For this review, use the dimensioned drawing (mm, ordinates from the lowest corner) and the shaded views. A direction names the side the tool comes from. Give positions to 0.01 mm unless a question says otherwise; leave off trailing zeros. Order: outer loops, then holes, each group sorted by start corner. A loop starts at its lowest first (then second) coordinate and runs counter-clockwise, first axis right, second up. Notation, with made-up numbers: M 20,55 L 47,55 A17 cw 47,77 Z; hole C 59.25,0.5 d3. An arc over 180 degrees is marked long. Answer as CSV lines item,"result". Start each with the question number.
1. We need section D-D, the plane y = 8. Give the boundary of the cut face in (x, z).
2. Clearance check with flat-ended pins moving along their axes: P1, Ø2, axis at x = 8, z = 16, coming from the -Y side; P2, Ø2, axis at y = 7.5, z = 30, coming from the -X side; P3, Ø1.5, axis at x = 3.5, z = 27.5, coming from the -Y side. State where each tip first meets the part, or that it passes through.
3. We need section C-C, the plane z = 19. Give the boundary of the cut face in (x, y).
4. For line 1 along Z through (x, y) = (6.5, 5); line 2 along Z through (x, y) = (1, 3.5); line 3 along X through (y, z) = (8.5, 22.5), list the stretches that pass through material, from the lowest coordinate up.
5. We need section A-A, the plane y = 5. Give the boundary of the cut face in (x, z), and give its area (3 significant figures).
6. Machinability: for the marked faces 1 and 2, which of the approach directions +Z, -Z, +X, -X, +Y, -Y give a long, thin tool a straight path to every point of the face, cutting with its end or side? Answer none if there is none.
7. We need section B-B, the plane x = 5. Give the boundary of the cut face in (y, z).
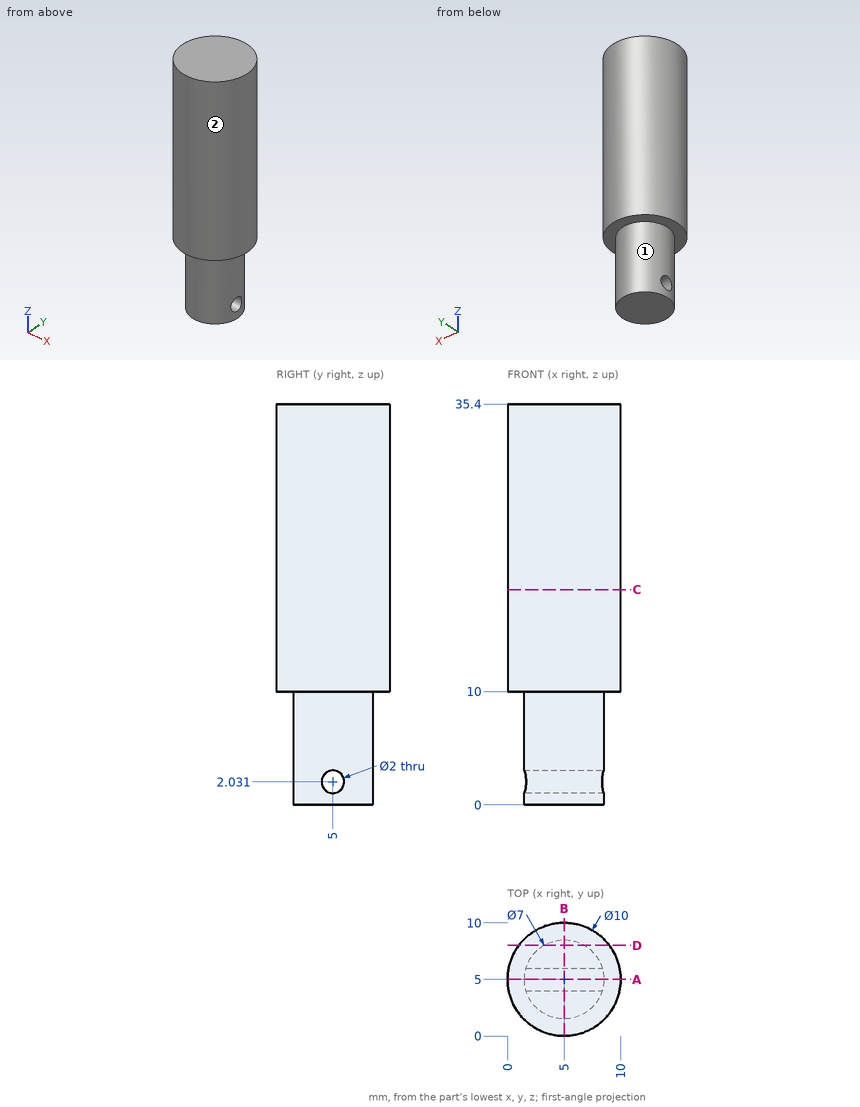
Result set:
1,outline,"M 1,10 L 3.2,10 L 3.2,0 L 6.8,0 L 6.8,10 L 9,10 L 9,35.4 L 1,35.4 Z"
2,P1,"y = 0.42"
2,P2,"x = 0.23"
2,P3,"y = 0.06"
3,outline,"C 5,5 d10"
4,line 1,"0 to 1.03, 3.03 to 35.4"
4,line 2,"10 to 35.4"
4,line 3,"1.43 to 8.57"
5,outline,"M 0,10 L 1.5,10 L 1.5,3.03 L 8.5,3.03 L 8.5,10 L 10,10 L 10,35.4 L 0,35.4 Z; M 1.5,0 L 8.5,0 L 8.5,1.03 L 1.5,1.03 Z"
5,area,"310 mm2"
6,face 1,"-Z"
6,face 2,"+Z, -Z"
7,outline,"M 0,10 L 1.5,10 L 1.5,0 L 8.5,0 L 8.5,10 L 10,10 L 10,35.4 L 0,35.4 Z; hole C 5,2.03 d2"
